Build history of the part. All positions in model axes, mm. A direction names the side the tool comes from. Round coordinates to 2 decimals unless told otherwise and drop trailing zeros. Use a Markdown table: item, result.
Autodesk Inventor part; units mm, degrees
ref_plane "YZ Plane" through (0, 0, 0) normal (1, 0, 0) x (0, 1, 0)
ref_plane "XZ Plane" through (0, 0, 0) normal (0, 1, 0) x (-1, 0, 0)
ref_plane "XY Plane" through (0, 0, 0) normal (0, 0, 1) x (1, 0, 0)
sketch "Sketch1" plane through (0, 0, 0) normal (1, 0, 0) x (0, 1, 0)
  circle A0 centre (-479.4213, -671.0964) radius 25.4
  circle A1 centre (-479.4213, -671.0964) radius 88.9
  circle A2 centre (-479.4213, -649.9452) radius 1.5875
  circle A3 centre (-497.7388, -660.5208) radius 1.5875
  circle A4 centre (-497.7388, -681.6721) radius 1.5875
  circle A5 centre (-479.4213, -692.2477) radius 1.5875
  circle A6 centre (-461.1038, -681.6721) radius 1.5875
  circle A7 centre (-461.1038, -660.5208) radius 1.5875
  point P0 (0, 0)
  dimension "d0" = 50.8
  dimension "d1" = 3.175
  dimension "d4" = 360
extrude "Extrusion1" add sketch "Sketch1" along normal blind 6.35 contours A0
sketch "Sketch2" plane through (6.35, -479.4213, -671.0964) normal (1, 0, 0) x (0, 0, -1)
  circle A0 centre (-21.1512, 0) radius 1.5875
  spline S0 degree 3 poles (-5.6187, -9.891) (-73.0206, -34.6538) (-119.0516, 78.5765) (-145.3355, 88.8855) knots 0 0 0 0 1 1 1 1
  spline S1 degree 3 poles (0, 11.5539) (-60.9983, -36.2975) (-102.9311, 114.869) (-133.6383, 103.832) knots 0 0 0 0 1 1 1 1
  line L0 (-145.3355, 88.8855) -> (-133.6383, 103.832)
  arc A1 (-5.6187, -9.891) -> (0, 11.5539) centre (0.2097, 0.0404) ccw
  point P0 (-671.0964, 479.4213)
  point P1 (-69.3034, 5.0557)
  point P2 (-121.2912, 64.8414)
  point P3 (-55.007, 16.7301)
  point P4 (-109.594, 88.8855)
extrude "Extrusion2" add sketch "Sketch2" along normal blind 19.05
sketch "Sketch3" plane through (6.35, -479.4213, -671.0964) normal (-1, 0, 0) x (0, 0, 1)
  spline S0 degree 3 poles (21.6253, -13.3232) (80.3701, -16.9336) (121.1871, 79.4141) (145.3355, 88.8855) knots 0 0 0 0 1 1 1 1
  line L0 (145.3355, 88.8855) -> (133.6383, 103.832)
  spline S1 degree 3 poles (133.6383, 103.832) (107.3744, 113.2719) (72.8986, 4.0539) (25.3056, 2.1884) knots 0 0 0 0 1 1 1 1
  line L1 (135.1558, 81.2846) -> (120.3749, 100.1713)
  point P0 (671.0964, 479.4213)
extrude "Extrusion3" add sketch "Sketch3" along normal blind 50.8
sketch "Sketch4" plane through (-44.45, -375.5893, -537.4582) normal (0, 0.6163082, 0.787505) x (1, 0, 0)
  line L0 (50.8, -18.9795) -> (0, -18.9795)
  spline S0 degree 4 poles (22.0839, 128.199) (22.0839, 128.1731) (22.0839, 75.9092) (22.0839, -57.7492) (22.0839, -145.2754) (22.0839, -219.2952) (22.0839, -161.3853) (22.0839, -142.8391) knots 0 0 0 0 0 0.294993 0.49649 0.669634 1 1 1 1 1
  spline S1 degree 4 poles (-3.3161, -142.8391) (-3.3161, -161.3853) (-3.3161, -219.2952) (-3.3161, -145.2754) (-3.3161, -57.7492) (-3.3161, 75.9092) (-3.3161, 128.1731) (-3.3161, 128.199) knots -1 -1 -1 -1 -1 -0.669634 -0.49649 -0.294993 0 0 0 0 0
  line L1 (-3.3161, 128.199) -> (22.0839, 128.199) construction
  line L2 (9.3839, 128.199) -> (9.3839, -142.8391) construction
  circle A0 centre (9.3839, -9.4897) radius 6.35
  point P0 (44.45, -35.4614)
  dimension "d12" = 12.7
extrude "Extrusion4" cut sketch "Sketch4" against normal through all
properties part number "fork"
Q1. Drill centre lines: L1, parallel to X at y = -436.5, z = -572.5; L2, parallel to Y at x = 11.5, z = -639.5; L3, parallel to Z at x = 8.5, y = -451. Where is each one in solid material? Low to high.
Response values:
| item | result |
|---|---|
| L1 | x = 6.35 to 25.4 |
| L2 | y = -492.41 to -476.36 |
| L3 | z = -604.92 to -578.4 |
Q2. Two-plate mould, pull along Z, no slides. Class faces 1 (the flat face through (-44.45, -386, -538)), 2 (the flat face through (6.35, -474, -682)), 3 (the cylindrical face through (3.13, -484.93, -646.3)): +Z half, -Z half, draft (parallel to the pull), parting line (faces both ways), or undercut.
Response values:
| item | result |
|---|---|
| face 1 | draft |
| face 2 | undercut |
| face 3 | parting line |
Q3. Drop flat-ended pins along their axis: P1, Ø3.5, axis at y = -497.74, z = -660.52, coming from the +X side; P2, Ø2, axis at x = 17.5, z = -547.5, coming from the +Y side; P3, Ø3.5, axis at y = -461.1, z = -681.67, coming from the -X side; P4, Ø12, axis at y = -430.5, z = -550, coming from the +X side. Give the stop position or say it passes through.
Response values:
| item | result |
|---|---|
| P1 | stops at x = 6.35 |
| P2 | stops at y = -376.52 |
| P3 | stops at x = 0 |
| P4 | passes through |
Q4. Which spindle directions (+Z, -Z, +X, -X, +Y, -Y) get a long thin tool onto all of the face, cutting with end or side? Do faces 4 (the flat face through (-18.694, -388.826, -543.228)), 5 (the flat face through (0, -480, -671)). Say none if no direction does.
Response values:
| item | result |
|---|---|
| face 4 | -Z, -X, -Y |
| face 5 | +Z, -Z, -X, +Y, -Y |
